from build123d import *

# Parameters (mm, degrees)
SKETCH_1_R          = 17
EXTRUDE_1_DEPTH     = 8
SKETCH_3_W          = 30
SKETCH_3_H          = 34
EXTRUDE_2_DEPTH     = 8
SKETCH_2_R          = 12.75
CUT_EXTRUDE_1_DEPTH = 8
SKETCH_4_W          = 19.904573782
SKETCH_4_H          = 25.5
CUT_EXTRUDE_2_DEPTH = 8


with BuildPart() as part:
    # 스케치1 → 보스-돌출1 (new body)
    with BuildSketch(Plane.XY):
        Circle(SKETCH_1_R)
    extrude(amount=EXTRUDE_1_DEPTH)

    # 스케치3 → 보스-돌출2 (add)
    with BuildSketch(Plane.XY.offset(8)):
        with Locations((3, 0)):
            Rectangle(SKETCH_3_W, SKETCH_3_H)
    extrude(amount=-EXTRUDE_2_DEPTH)

    # 스케치2 → 컷-돌출1 (cut)
    with BuildSketch(Plane.XY.offset(8)):
        Circle(SKETCH_2_R)
    extrude(amount=-CUT_EXTRUDE_1_DEPTH, mode=Mode.SUBTRACT)

    # 스케치4 → 컷-돌출2 (cut)
    with BuildSketch(Plane(origin=(0, 0, 0), x_dir=(-1, 0, 0), z_dir=(0, 0, -1))):
        with Locations((9.952286891, 0)):
            Rectangle(SKETCH_4_W, SKETCH_4_H)
    extrude(amount=-CUT_EXTRUDE_2_DEPTH, mode=Mode.SUBTRACT)


solid = part.part
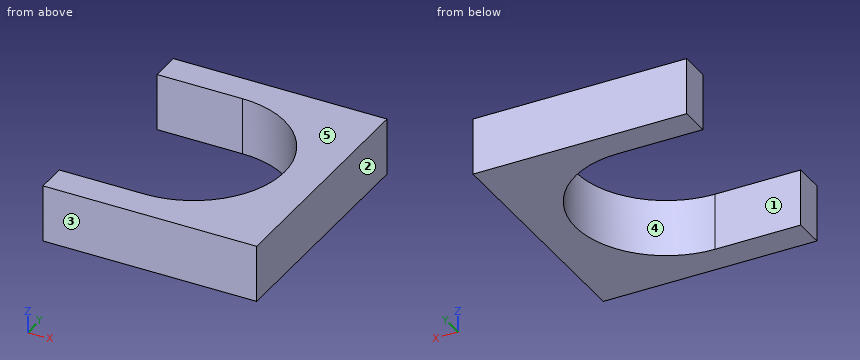
The listing builds one solid part. Answer for the finished solid, in the listing's coordinates (mm). Face numbers are marked on the shaded views. A direction names the side the tool comes from. Coordinates: 2 decimals unless noted, no trailing zeros. Loops run counter-clockwise (first coordinate to the right, second up) from the corner with the lowest first, then second, coordinate; pieces in that order, holes last. Notation, with made-up numbers: (33, 21) -> (37, 21) arc R3 cw to (37, 26) -> close; hole circle Ø1 at (-18, 38). An arc over 180 degrees is marked (long way). Write item = value, one per line. Start each with the question number.
1) The mould has two halves that part along Y. Classify the marked faces 3, 4 and 5: released by +Y, released by -Y, zero draft, split by the parting line, or undercut.
2) A cutting plane is placed at A-A (x = -4). Give the vertices of the cut face in (y, z), then the cut area to 3 significant figures.
3) A tool of negligible diameter and unlimited length cuts with its end or side. For the marked faces 1 and 2, from which of +Z, -Z, +X, -X, +Y, -Y can it reach the whole face along a straight path? Write none if from no direction.
4) A cutting plane is placed at B-B (z = 1.75). Give the vertices of the cut face in (x, y).
5) Straight lines are drawn through the part: line 1 (Y direction, x = -10.5, z = 7.5); line 2 (Y direction, x = 4.75, z = 1.75); line 3 (X direction, y = -11, z = 3.25). For each, find the intervals that lie inside material, in ascending order. Write a range as from..to.
6) A cutting plane is placed at D-D (x = 7). Give the vertices of the cut face in (y, z), then the cut area to 3 significant figures.
7) A cutting plane is placed at C-C (y = 0). Give the vertices of the cut face in (x, z).
8) Given pin 1 Ø2 at (x, y) = (12, -8.5) entering from -Z, flat-ended and moving along its own axis, determine where the tip first touches the part or whether it passes through.
Responses:
q1.face_3 = released by -Y
q1.face_4 = undercut
q1.face_5 = zero draft
q2.outline = (-17, 0) -> (-12.75, 0) -> (-12.75, 8) -> (-17, 8) -> close; (12.75, 0) -> (17, 0) -> (17, 8) -> (12.75, 8) -> close
q2.area = 68.0 mm²
q3.face_1 = +Z, -Z, -X
q3.face_2 = +Z, -Z, +X, +Y, -Y
q4.outline = (-12, -17) -> (18, -17) -> (18, 17) -> (-12, 17) -> (-12, 12.75) -> (0, 12.75) arc R12.75 cw to (0, -12.75) -> (-12, -12.75) -> close
q5.line_1 = -17..-12.75, 12.75..17
q5.line_2 = -17..-11.83, 11.83..17
q5.line_3 = 6.45..18
q6.outline = (-17, 0) -> (-10.66, 0) -> (-10.66, 8) -> (-17, 8) -> close; (10.66, 0) -> (17, 0) -> (17, 8) -> (10.66, 8) -> close
q6.area = 101 mm²
q7.outline = (12.75, 0) -> (18, 0) -> (18, 8) -> (12.75, 8) -> close
q8.pin_1 = 0
